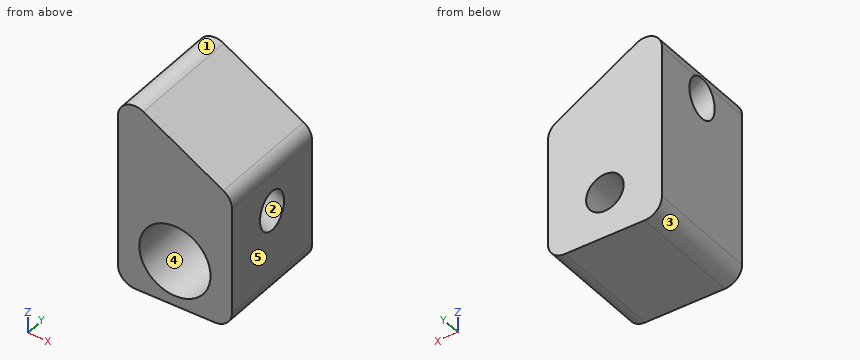
from build123d import *

# Parameters (mm, degrees)
F1_DEPTH       = 20
F5_D           = 6.6
F5_CBORE_D     = 12.5
F5_CBORE_DEPTH = 12
F7_T1_DEPTH    = 45.9807621135
F7_T3_DEPTH    = 28.6602540378
F7_T5_DEPTH    = 35


# Not quite as in the source:
# - a fillet or chamfer that OpenCascade refuses, or shapes differently, is made with other operations: its cross-section is extruded or revolved along the edge and cut away or added


with BuildPart() as f1:
    # F0 (on Front) → F1 (new body)
    with BuildSketch(Plane.XZ):
        Polygon((-10, -20), (10, -20), (10, 3.4529946162), (-10, 15), align=None)
    extrude(amount=F1_DEPTH)

    # F5 (through all)
    with Locations(Plane.XZ.offset(20)):
        with Locations((0, -12)):
            CounterBoreHole(F5_D / 2, F5_CBORE_D / 2, F5_CBORE_DEPTH)

    # F3 (on offset) → F6 (revolve, cut)
    with BuildSketch(Plane.XZ.offset(10)):
        Polygon((-10.3968404344, 10.6191993773), (-10.3968404344, 6.9818926814), (13.3675798804, -6.7385017846), (13.3675798804, -3.2744001694), (2.5, 3), (0, 3), (0.8023552889, 4.1533407117), align=None)
    revolve(axis=Axis((1.485369723, -10, 0.1216954484), (-0.8660254038, 0, 0.5)), mode=Mode.SUBTRACT)

    # F7: fillet of radius 3 on 4 edges, made by hand

    # F7_s2 → F7_t1 (cut)
    with BuildSketch(Plane.XZ.offset(-12.9903810568)):
        with BuildLine():
            ThreePointArc((-5.5, 12.4019237886), (-8.5, 12.4019237886), (-10, 9.8038475773))
            Line((-10, 9.8038475773), (-10, 15))
            Line((-10, 15), (-5.5, 12.4019237886))
        make_face()
    extrude(amount=F7_T1_DEPTH, mode=Mode.SUBTRACT)

    # F7_s4 → F7_t3 (cut)
    with BuildSketch(Plane.XZ.offset(-4.3301270189)):
        with BuildLine():
            ThreePointArc((8.5, 4.31902002), (9.5980762114, 3.2209438086), (10, 1.7209438086))
            Line((10, 1.7209438086), (10, 3.4529946162))
            Line((10, 3.4529946162), (8.5, 4.31902002))
        make_face()
    extrude(amount=F7_T3_DEPTH, mode=Mode.SUBTRACT)

    # F7_s6 → F7_t5 (cut)
    with BuildSketch(Plane.XZ.offset(-7.5)):
        with BuildLine():
            ThreePointArc((10, -17), (9.1213203436, -19.1213203436), (7, -20))
            Line((7, -20), (10, -20))
            Line((10, -20), (10, -17))
        make_face()
        with BuildLine():
            ThreePointArc((-10, -17), (-9.1213203436, -19.1213203436), (-7, -20))
            Line((-7, -20), (-10, -20))
            Line((-10, -20), (-10, -17))
        make_face()
    extrude(amount=F7_T5_DEPTH, mode=Mode.SUBTRACT)


solid = f1.part
Geometry: final body of the model. Coordinates: model frame, mm. Face numbers are marked on the shaded views. A direction names the side the tool comes from. Coordinates: 2 decimals unless noted, no trailing zeros. Loops run counter-clockwise (first coordinate to the right, second up) from the corner with the lowest first, then second, coordinate; pieces in that order, holes last. Notation, with made-up numbers: (-12.5, 0) - (9.5, 0) arc R16 ccw to (9.5, 8) - close; hole circle Ø7 at (-4.75, 72.5). An arc over 180 degrees is marked (long way). Put each result on its own line as item: value. Start each with the question number.
Q1. Line query: line 1 (Z direction, x = -4.75, y = -10.25); line 2 (Z direction, x = 1.25, y = -9); line 3 (X direction, y = -9.75, z = -11). Output: solid intervals per line, ascending.
Q2. Cut plane A-A, the plane z = -12. Return loops of the section in (x, y).
Q3. Pin query (flat end, axial travel): pin 1 Ø3 at (y, z) = (-6, 5.5) entering from +X; pin 2 Ø11 at (x, z) = (0, -12) entering from -Y; pin 3 Ø4 at (x, y) = (5, -6) entering from +Z. Return the tip coordinate at first contact, or that it passes through.
Q4. Cut plane D-D, the plane y = -16.25. Return loops of the section in (x, z).
Q5. Pull-direction query (Z, two-part tool) for the marked faces 1, 2 and 3; classes: released by +Z, released by -Z, zero draft, split by the parting line, or undercut.
Q6. Cut plane C-C, the plane x = -1. Give the number of separate pieces and of enclosed holes in the cut face, and give its area (3 significant figures).
Q7. Cut plane B-B, the plane y = -2.75. Return loops of the section in (x, z).
Q8. Set-up query: the marked faces 4 and 5. Return all of +Z, -Z, +X, -X, +Y, -Y with unobstructed straight access to the full face (end or side cutting, diameter ignored); none if empty.
Filled sheet:
1. line 1: -20 to -16.06, -7.94 to 0.1, 7.35 to 11.97
1. line 2: -20 to -18.12, -5.88 to -3.01, 2.81 to 8.5
1. line 3: -10 to -6.17, 6.17 to 10
2. outline: (-10, -20) - (-6.25, -20) - (-6.25, -8) - (-3.3, -8) - (-3.3, 0) - (-10, 0) - close; (3.3, -8) - (6.25, -8) - (6.25, -20) - (10, -20) - (10, 0) - (3.3, 0) - close
3. pin 1: x = 8.95
3. pin 2: y = -8
3. pin 3: z = 7.49
4. outline: (-10, -17) arc R3 ccw to (-7, -20) - (7, -20) arc R3 ccw to (10, -17) - (10, 1.72) arc R3 ccw to (8.5, 4.32) - (-5.5, 12.4) arc R3 ccw to (-10, 9.8) - close; hole circle Ø12.5 at (0, -12)
5. face 1: released by +Z
5. face 2: undercut
5. face 3: released by -Z
6. separate pieces: 2
6. enclosed holes: 1
6. area: 370 mm²
7. outline: (-10, -17) arc R3 ccw to (-7, -20) - (7, -20) arc R3 ccw to (10, -17) - (10, 1.72) arc R3 ccw to (8.5, 4.32) - (-5.5, 12.4) arc R3 ccw to (-10, 9.8) - close; hole circle Ø6.6 at (0, -12)
8. face 4: -Y
8. face 5: +Z, -Z, +X, +Y, -Y
